Check sheet for the modelled part. Datum: model origin and axes. Units: mm. Face numbers are marked on the shaded views. Round coordinates to 2 decimals unless told otherwise and drop trailing zeros. Loops run counter-clockwise (first coordinate to the right, second up) from the corner with the lowest first, then second, coordinate; pieces in that order, holes last. Notation, with made-up numbers: (31.25, 47.25) - (52.25, 47.25) arc R26 ccw to (52.25, 68.25) - close; hole circle Ø8 at (88.5, 86). An arc over 180 degrees is marked (long way). Answer in a Markdown table with one row per item. Add a question column.
(1) Cross-section at C-C on y = 1.25. Enter the section's corners in (x, z), then the cut area to 3 significant figures.
(2) Mould release check, pull along Z, two halves, no side actions. Record for the marked faces 1, 2 and 3: +Z half, -Z half, draft (parallel to the pull), parting line (faces both ways), or undercut.
(3) Cross-section at D-D on z = 2.75. Enter the section's corners in (x, y), then the cut area to 3 significant figures.
(4) Cross-section at B-B on x = 0. Enter the section's corners in (y, z), then the cut area to 3 significant figures.
(5) Thickness scan on line 1 along Z through (x, y) = (0, 2.25); line 2 along X through (y, z) = (-0.5, 8.5); line 3 along Z through (x, y) = (6.5, -0.5). Record the ranges inside material, lowest first.
(6) Cross-section at A-A on z = 8.5. Enter the section's corners in (x, y), then the cut area to 3 significant figures.
(7) Gauge pin test, flat end, axial feed: pin 1 (1.3 mm diameter, centred on x = -1.5, z = -1, fed in from -Y). Record the tip position at first contact, or that the pin passes through.
from build123d import *

# Parameters (mm, degrees)
SKETCH1_W           = 18
SKETCH1_H           = 10
BOSS_EXTRUDE1_DEPTH = 16
SKETCH6_R           = 6
CUT_EXTRUDE1_DEPTH  = 11
BOSS_EXTRUDE2_DEPTH = 8


with BuildPart() as part:
    # Sketch1 → Boss-Extrude1 (new body)
    with BuildSketch(Plane.XY):
        Rectangle(SKETCH1_W, SKETCH1_H)
    extrude(amount=BOSS_EXTRUDE1_DEPTH)

    # Sketch6 → Cut-Extrude1 (cut, through all)
    with BuildSketch(Plane(origin=(0, 5, 0), x_dir=(1, 0, 0), z_dir=(0, 1, 0))):
        with Locations((0, -8.5)):
            Circle(SKETCH6_R)
    extrude(amount=-CUT_EXTRUDE1_DEPTH, mode=Mode.SUBTRACT)

    # Sketch8 → Boss-Extrude2 (add)
    with BuildSketch(Plane(origin=(0, 5, 0), x_dir=(1, 0, 0), z_dir=(0, 1, 0))):
        Polygon((-1.45, 0), (-2.95, 2.598076211), (2.95, 2.598076211), (1.45, 0), align=None)
    extrude(amount=-BOSS_EXTRUDE2_DEPTH)


solid = part.part
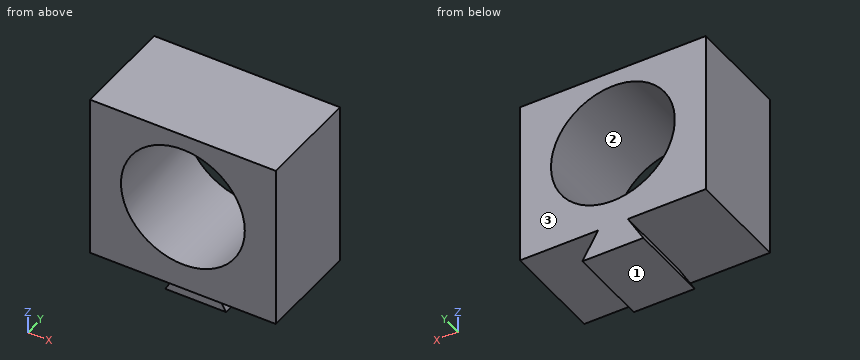
Answers:
| question | item | result |
|---|---|---|
| 1 | outline | (-9, 0) - (-1.45, 0) - (-2.95, -2.6) - (2.95, -2.6) - (1.45, 0) - (9, 0) - (9, 16) - (-9, 16) - close; hole circle Ø12 at (0, 8.5) |
| 1 | area | 186 mm^2 |
| 2 | face 1 | -Z half |
| 2 | face 2 | undercut |
| 2 | face 3 | draft |
| 3 | outline | (-9, -5) - (-1.71, -5) - (-1.71, 5) - (-9, 5) - close; (1.71, -5) - (9, -5) - (9, 5) - (1.71, 5) - close |
| 3 | area | 146 mm^2 |
| 4 | outline | (-5, 0) - (-3, 0) - (-3, -2.6) - (5, -2.6) - (5, 2.5) - (-5, 2.5) - close; (-5, 14.5) - (5, 14.5) - (5, 16) - (-5, 16) - close |
| 4 | area | 60.8 mm^2 |
| 5 | line 1 | z = -2.6 to 2.5, 14.5 to 16 |
| 5 | line 2 | x = -9 to -6, 6 to 9 |
| 5 | line 3 | z = 0 to 16 |
| 6 | outline | (-9, -5) - (-6, -5) - (-6, 5) - (-9, 5) - close; (6, -5) - (9, -5) - (9, 5) - (6, 5) - close |
| 6 | area | 60.0 mm^2 |
| 7 | pin 1 | stops at y = -3 |
